```python
from build123d import *

# Parameters (mm, degrees)
SKETCH1_W           = 145
SKETCH1_H           = 43
SKETCH1_R           = 1.5875
BOSS_EXTRUDE1_DEPTH = 3
SKETCH4_W           = 10
SKETCH4_H           = 8
BOSS_EXTRUDE3_DEPTH = 10
CHAMFER2_SIZE       = 5
SKETCH5_R           = 2.2
CUT_EXTRUDE2_DEPTH  = 5.2


with BuildPart() as part:
    # Sketch1 → Boss-Extrude1 (new body)
    with BuildSketch(Plane(origin=(0, 0, 0), x_dir=(1, 0, 0), z_dir=(0, 1, 0))):
        Rectangle(SKETCH1_W, SKETCH1_H)
        with Locations(Location((-57.8125, 15.621, 0), (0, 0, 270))):
            Circle(SKETCH1_R, mode=Mode.SUBTRACT)
        with Locations(Location((-45.1125, 15.621, 0), (0, 0, 270))):
            Circle(SKETCH1_R, mode=Mode.SUBTRACT)
        with Locations(Location((-26.0625, 15.621, 0), (0, 0, 270))):
            Circle(SKETCH1_R, mode=Mode.SUBTRACT)
        with Locations(Location((-26.0625, -15.621, 0), (0, 0, 270))):
            Circle(SKETCH1_R, mode=Mode.SUBTRACT)
        with Locations(Location((-45.1125, -15.621, 0), (0, 0, 270))):
            Circle(SKETCH1_R, mode=Mode.SUBTRACT)
        with Locations(Location((-57.8125, -15.621, 0), (0, 0, 270))):
            Circle(SKETCH1_R, mode=Mode.SUBTRACT)
        with Locations(Location((45.1125, -15.621, 0), (0, 0, 90))):
            Circle(SKETCH1_R, mode=Mode.SUBTRACT)
        with Locations(Location((26.0625, -15.621, 0), (0, 0, 90))):
            Circle(SKETCH1_R, mode=Mode.SUBTRACT)
        with Locations(Location((26.0625, 15.621, 0), (0, 0, 90))):
            Circle(SKETCH1_R, mode=Mode.SUBTRACT)
        with Locations(Location((45.1125, 15.621, 0), (0, 0, 90))):
            Circle(SKETCH1_R, mode=Mode.SUBTRACT)
        with Locations(Location((57.8125, 15.621, 0), (0, 0, 90))):
            Circle(SKETCH1_R, mode=Mode.SUBTRACT)
        with Locations(Location((57.8125, -15.621, 0), (0, 0, 90))):
            Circle(SKETCH1_R, mode=Mode.SUBTRACT)
    extrude(amount=BOSS_EXTRUDE1_DEPTH)

    # Sketch4 → Boss-Extrude3 (add)
    with BuildSketch(Plane(origin=(0, 3, 0), x_dir=(1, 0, 0), z_dir=(0, 1, 0))):
        with Locations((-35.5875, 17.5)):
            Rectangle(SKETCH4_W, SKETCH4_H)
        with Locations((35.5875, 17.5)):
            Rectangle(SKETCH4_W, SKETCH4_H)
    extrude(amount=BOSS_EXTRUDE3_DEPTH)

    # Chamfer2
    chamfer2_edges = [part.edges().sort_by_distance(p)[0] for p in [
        (-35.5875, 3, -13.5),
        (35.5875, 3, -13.5),
    ]]
    chamfer(chamfer2_edges, length=CHAMFER2_SIZE)

    # Sketch5 → Cut-Extrude2 (cut)
    with BuildSketch(Plane(origin=(0, 0, -21.5), x_dir=(-1, 0, 0), z_dir=(0, 0, -1))):
        with Locations((-35.5875, 6.5)):
            Circle(SKETCH5_R)
        with Locations((35.5875, 6.5)):
            Circle(SKETCH5_R)
    extrude(amount=-CUT_EXTRUDE2_DEPTH, mode=Mode.SUBTRACT)


solid = part.part
```
The model under review builds one solid part; all positions refer to its coordinate system, in mm. A direction names the side the tool comes from. Round coordinates to 2 decimals unless told otherwise and drop trailing zeros. Write each loop counter-clockwise with the first axis right and the second up, starting at its lowest first coordinate (ties: lowest second). Pieces come first, ordered by that corner, then holes. Notation, with made-up numbers: M 26.25,-30.75 L 84.25,-30.75 A19 ccw 84.25,-20.75 Z; hole C 25,-14.75 d9. An arc over 180 degrees is marked long. Use CSV: the item, a comma, the result in double quotes. Start each with the question number.
(1) For line 1 along Z through (x, y) = (-27.5, 1.25); line 2 along Y through (x, z) = (-57, 18); line 3 along Z through (x, y) = (38.5, 8.5), list the stretches that pass through material, from the lowest coordinate up.
(2) Tool access review of faces 4 (the face through (40.588, 7, -16)), 5 (the face through (36, 10, -13.5)), 6 (the face through (36, 7, -16.3)), 7 (the face through (-27.61, 1.48, -15.97)), 8 (the face through (-30.588, 7, -16)): name each direction out of +Z, -Z, +X, -X, +Y, -Y from which nothing blocks a thin tool from reaching the whole face with its end or side.
(3) We need section D-D, the plane x = 42. State the section outline as (y, z) points.
(4) We need section B-B, the plane z = -11. State the section outline as (x, y) points, then the cut area to 3 significant figures.
(5) The part is to be moulded in two halves that separate along X. For faces 1 (the face through (-35.7, 5.5, -11)), 2 (the face through (46.662, 1.479, -15.277)), 3 (the face through (-40.588, 7, -16)), say which applies: +X half, -X half, draft (parallel to the pull), parting line (faces both ways), or undercut.
(6) Clearance check with flat-ended pins moving along their axes: P1, Ø3, axis at y = 6, z = -17.5, coming from the +X side; P2, Ø3, axis at y = 5.5, z = -17.5, coming from the -X side; P3, Ø4, axis at x = 45.11, z = -15.62, coming from the +Y side. State where each tip first meets the part, or that it passes through.
(7) We need section A-A, the plane y = 6.5. State the section outline as (x, z) points.
(8) We need section C-C, the plane z = 15.5. State the section outline as (x, y) points.
Findings:
1,line 1,"-21.5 to -16.29, -14.95 to 14.95, 16.29 to 21.5"
1,line 2,"0 to 3"
1,line 3,"-21.5 to -13.5"
2,face 4,"+Z, -Z, +X, +Y"
2,face 5,"+Z, +X, -X, +Y"
2,face 6,"-Z"
2,face 7,"+Y, -Y"
2,face 8,"+Z, -Z, +Y"
3,outline,"M 0,-21.5 L 3,-21.5 L 3,21.5 L 0,21.5 Z"
4,outline,"M -72.5,0 L 72.5,0 L 72.5,3 L 40.59,3 L 40.59,5.5 L 30.59,5.5 L 30.59,3 L -30.59,3 L -30.59,5.5 L -40.59,5.5 L -40.59,3 L -72.5,3 Z"
4,area,"485 mm^2"
5,face 1,"draft"
5,face 2,"undercut"
5,face 3,"-X half"
6,P1,"x = 40.59"
6,P2,"x = -40.59"
6,P3,"y = 3"
7,outline,"M -40.59,-21.5 L -37.79,-21.5 L -37.79,-16.3 L -33.39,-16.3 L -33.39,-21.5 L -30.59,-21.5 L -30.59,-12 L -40.59,-12 Z; M 30.59,-21.5 L 33.39,-21.5 L 33.39,-16.3 L 37.79,-16.3 L 37.79,-21.5 L 40.59,-21.5 L 40.59,-12 L 30.59,-12 Z"
8,outline,"M -72.5,0 L -59.4,0 L -59.4,3 L -72.5,3 Z; M -56.23,0 L -46.7,0 L -46.7,3 L -56.23,3 Z; M -43.53,0 L -27.65,0 L -27.65,3 L -43.53,3 Z; M -24.48,0 L 24.48,0 L 24.48,3 L -24.48,3 Z; M 27.65,0 L 43.53,0 L 43.53,3 L 27.65,3 Z; M 46.7,0 L 56.23,0 L 56.23,3 L 46.7,3 Z; M 59.4,0 L 72.5,0 L 72.5,3 L 59.4,3 Z"
